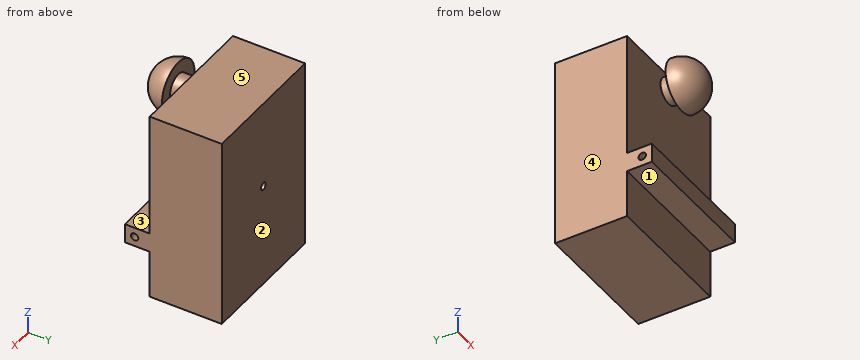
```python
from build123d import *

# Parameters (mm, degrees)
SKETCH2_W           = 180
SKETCH2_H           = 259.71
BOSS_EXTRUDE1_DEPTH = 97.5
SKETCH4_R           = 17.7
BOSS_EXTRUDE2_DEPTH = 17.7
SKETCH5_R           = 35
BOSS_EXTRUDE3_DEPTH = 35
FILLET2_R           = 35
SKETCH8_W           = 180
SKETCH8_H           = 26.2
BOSS_EXTRUDE4_DEPTH = 33.5
SKETCH9_R           = 5
CUT_EXTRUDE1_DEPTH  = 250.575830668
SKETCH10_R          = 5
CUT_EXTRUDE2_DEPTH  = 10


with BuildPart() as part:
    # Sketch2 → Boss-Extrude1 (new body)
    with BuildSketch(Plane(origin=(0, 0, 0), x_dir=(1, 0, 0), z_dir=(0, 1, 0))):
        Rectangle(SKETCH2_W, SKETCH2_H)
    extrude(amount=BOSS_EXTRUDE1_DEPTH)

    # Sketch4 → Boss-Extrude2 (add)
    with BuildSketch(Plane.XZ):
        with Locations(Location((0, 107.765, 0), (0, 0, 270))):
            Circle(SKETCH4_R)
    extrude(amount=BOSS_EXTRUDE2_DEPTH)

    # Sketch5 → Boss-Extrude3 (add)
    with BuildSketch(Plane.XZ.offset(17.7)):
        with Locations(Location((0, 107.765, 0), (0, 0, 270))):
            Circle(SKETCH5_R)
    extrude(amount=BOSS_EXTRUDE3_DEPTH)

    # Fillet2
    fillet2_edges = [part.edges().sort_by_distance(p)[0] for p in [
        (0, -52.7, 142.765),
    ]]
    fillet(fillet2_edges, radius=FILLET2_R - 0.0001)  # a hair under: the kernel refuses the full size

    # Sketch8 → Boss-Extrude4 (add)
    with BuildSketch(Plane.XZ):
        with Locations((0, -51.935)):
            Rectangle(SKETCH8_W, SKETCH8_H)
    extrude(amount=BOSS_EXTRUDE4_DEPTH)

    # Sketch9 → Cut-Extrude1 (cut, through all)
    with BuildSketch(Plane(origin=(90, 0, 0), x_dir=(0, 0, -1), z_dir=(1, 0, 0))):
        with Locations((51.935, -20.5)):
            Circle(SKETCH9_R)
    extrude(amount=-CUT_EXTRUDE1_DEPTH, mode=Mode.SUBTRACT)

    # Sketch10 → Cut-Extrude2 (cut)
    with BuildSketch(Plane(origin=(0, 97.5, 0), x_dir=(1, 0, 0), z_dir=(0, 1, 0))):
        with Locations(Location((0, -10.705, 0), (0, 0, 270))):
            Circle(SKETCH10_R)
    extrude(amount=-CUT_EXTRUDE2_DEPTH, mode=Mode.SUBTRACT)


solid = part.part
```
Can you work these out from the model? Positions are in its coordinate system, mm. Face numbers are marked on the shaded views. A direction names the side the tool comes from. Round coordinates to 2 decimals unless told otherwise and drop trailing zeros. Order: outer loops, then holes, each group sorted by start corner. A loop starts at its lowest first (then second) coordinate and runs counter-clockwise, first axis right, second up. Notation, with made-up numbers: (46.25, 75.5) -> (91.25, 75.5) arc R33 ccw to (91.25, 108.5) -> close; hole circle Ø7 at (46, 53). An arc over 180 degrees is marked (long way). Return JSON: item names as keys, results as strings. Group by question number.
1. Will these pins go through, and if not, where does the flat tip stop? pin 1 (17 mm diameter, centred on x = 19, y = -16.5, fed in from -Z) (3 decimals); pin 2 (4 mm diameter, centred on x = -68, y = 43.5, fed in from +Z) (3 decimals); pin 3 (4 mm diameter, centred on x = -24.5, z = 19, fed in from -Y).
2. I need wall thicknesses on line 1 (Y direction, x = -48.5, z = -86); line 2 (Z direction, x = 60.5, y = 77.5) (3 decimals); line 3 (Z direction, x = -62, y = -25) (3 decimals). Which ranges of each line are inside material? Lowest first, please. Write a range as [from, to].
3. Which directions (+Z, -Z, +X, -X, +Y, -Y) give clear straight access to the entire face, cutting with the end or side of a thin tool? Please do the marked faces 1, 2, 3, 4 and 5.
4. If we section it at B-B, the plane z = 46: Write out the boundary of the cut face in (x, y), then the cut area to 4 significant figures.
5. If we section it at A-A, the plane y = 61: Write out the boundary of the cut face in (x, z) (3 decimals), then the cut area to 3 significant figures.
Output values:
{
 "1": {"pin 1": "z = -65.035", "pin 2": "z = 129.855", "pin 3": "y = 0"},
 "2": {"line 1": "[0, 97.5]", "line 2": "[-129.855, 129.855]", "line 3": "[-65.035, -54.114], [-49.756, -38.835]"},
 "3": {"face 1": "-Z, +X, -X, -Y", "face 2": "+Z, -Z, +X, -X, +Y", "face 3": "+X, -X, -Y", "face 4": "+Z, -Z, -X, +Y, -Y", "face 5": "+Z, +X, -X, +Y"},
 "4": {"outline": "(-90, 0) -> (90, 0) -> (90, 97.5) -> (-90, 97.5) -> close", "area": "17,550 mm²"},
 "5": {"outline": "(-90, -129.855) -> (90, -129.855) -> (90, 129.855) -> (-90, 129.855) -> close", "area": "46,700 mm²"}
}
